Can you work these out from the model? Positions are in its coordinate system, mm. Face numbers are marked on the shaded views. A direction names the side the tool comes from. Round coordinates to 2 decimals unless told otherwise and drop trailing zeros. Loops run counter-clockwise (first coordinate to the right, second up) from the corner with the lowest first, then second, coordinate; pieces in that order, holes last. Notation, with made-up numbers: M 83,87 L 89,87 A19 cw 89,102 Z; hole C -2,32 d10. An arc over 180 degrees is marked long. Return JSON: item names as keys, results as strings.
```python
from build123d import *

# Parameters (mm, degrees)
F1_DEPTH = 5
F2_SIZE  = 4.99999
F4_DEPTH = 2.5


# Not quite as in the source:
# - a fillet or chamfer is up to 0.001 mm smaller than in the source, because OpenCascade refuses the exact size


with BuildPart() as f1:
    # F0 (on Top) → F1 (new body)
    with BuildSketch(Plane.XY):
        Polygon((-35, -47.5), (35, -47.5), (35, -11.5), (24.9973740429, 8.3822524399), (14.7012080997, -26.056649141), (0, 0), (-10.1515629949, -11.1895798258), (-20.0927332044, 15.4384202456), (-35, -14.74), align=None)
        Polygon((35, -11.5), (35, -47.5), (-35, -47.5), (-35, -14.74), (-40, -14.74), (-40, -52.5), (40, -52.5), (40, -11.5), align=None)
    extrude(amount=F1_DEPTH)

    # F2 (size 5 in the source; OpenCascade refuses exactly that, so slightly less here)
    f2_edges = [f1.edges().sort_by_distance(p)[0] for p in [
        (40, -32, 0),
        (0, -52.5, 0),
        (-40, -33.62, 0),
    ]]
    chamfer(f2_edges, length=F2_SIZE)

    # F3 (on face) → F4 (join)
    with BuildSketch(Plane(origin=(0, 0, 0), x_dir=(1, 0, 0), z_dir=(0, 0, -1))):
        with BuildLine():
            ThreePointArc((-33.1967424913, 11.0894674339), (-34.5462442763, 5.6175623185), (-35, 0))
            ThreePointArc((-35, 0), (0, -35), (35, 0))
            ThreePointArc((35, 0), (34.6974429309, 4.5921078013), (33.7950026252, 9.1048227638))
            Line((33.7950026252, 9.1048227638), (24.9973740429, -8.3822524399))
            Line((24.9973740429, -8.3822524399), (18.0845360262, 14.74))
            Line((18.0845360262, 14.74), (8.3163343919, 14.74))
            Line((8.3163343919, 14.74), (0, 0))
            Line((0, 0), (-10.1515629949, 11.1895798258))
            Line((-10.1515629949, 11.1895798258), (-20.0927332044, -15.4384202456))
            Line((-20.0927332044, -15.4384202456), (-33.1967424913, 11.0894674339))
        make_face()
        Polygon((14.7012080997, 26.056649141), (8.3163343919, 14.74), (18.0845360262, 14.74), align=None)
        with BuildLine():
            Line((-35, 14.74), (-35, 0))
            ThreePointArc((-35, 0), (-34.5462442763, 5.6175623185), (-33.1967424913, 11.0894674339))
            Line((-33.1967424913, 11.0894674339), (-35, 14.74))
        make_face()
        with BuildLine():
            ThreePointArc((33.7950026252, 9.1048227638), (34.6974429309, 4.5921078013), (35, 0))
            Line((35, 0), (35, 11.5))
            Line((35, 11.5), (33.7950026252, 9.1048227638))
        make_face()
    extrude(amount=-F4_DEPTH)


solid = f1.part
```
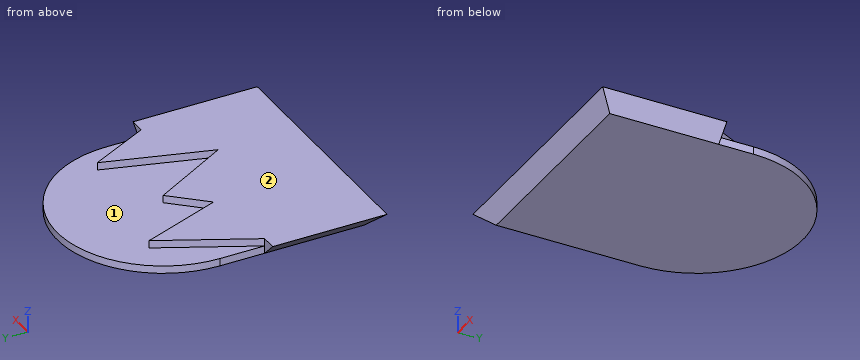
Q1. Suppose I cut it at B-B, the plane z = 4.2. Please give me the cut outline in (x, y), plus the area to 3 significant figures.
Results:
{"outline": "M -39.2,-51.7 L 39.2,-51.7 L 39.2,-11.5 L 35,-11.5 L 25,8.38 L 14.7,-26.06 L 0,0 L -10.15,-11.19 L -20.09,15.44 L -35,-14.74 L -39.2,-14.74 Z", "area": "3,610 mm2"}
Q2. Suppose I cut it at C-C, the plane y = 27.5. Please give me the cut outline in (x, z).
Results:
{"outline": "M -21.65,0 L 21.65,0 L 21.65,2.5 L -21.65,2.5 Z"}
Q3. If I drill on line 1 along Z through (x, y) = (16, 2); line 2 along Y through (x, z) = (-14.5, 2.05); line 3 along X through (y, z) = (-35.5, 1.5), over which ranges is the centre line in solid material (lowest first)?
Results:
{"line 1": "z = 0 to 2.5", "line 2": "y = -49.55 to 31.86", "line 3": "x = -36.5 to 36.5"}
Q4. I'm going to push flat-ended pins straight in: pin 1 Ø2.5 at (x, z) = (37, 2.5) entering from +Y; pin 2 Ø0.8 at (y, z) = (-9.5, 1) entering from -X; pin 3 Ø3 at (x, z) = (-22.5, 1.5) entering from +Y; pin 4 Ø6 at (x, y) = (27, -33.5) entering from -Z. Where does each tip first touch, or does it pass through?
Results:
{"pin 1": "stops at y = -11.5", "pin 2": "stops at x = -35", "pin 3": "stops at y = 28", "pin 4": "stops at z = 0"}
Q5. On a 3-axis mill with a long thin cutter (end or side, diameter ignored), from which of +Z, -Z, +X, -X, +Y, -Y can I reach the whole of each face in a straight line? I mean the marked faces 1 and 2. Say none if no direction works.
Results:
{"face 1": "+Z, +Y", "face 2": "+Z, +X, -X, +Y, -Y"}
